Geometry: see drawing. Coordinates: mm, zero at the bounding-box minimum. A direction names the side the tool comes from. Round coordinates to 2 decimals unless told otherwise and drop trailing zeros. Write each loop counter-clockwise with the first axis right and the second up, starting at its lowest first coordinate (ties: lowest second). Pieces come first, ordered by that corner, then holes. Notation, with made-up numbers: M 0,-11 L 58,-11 A23 cw 58,15 Z; hole C 55,16 d3. An arc over 180 degrees is marked long. Write each question's results on one line, items separated by ' | '. Start each with the question number.
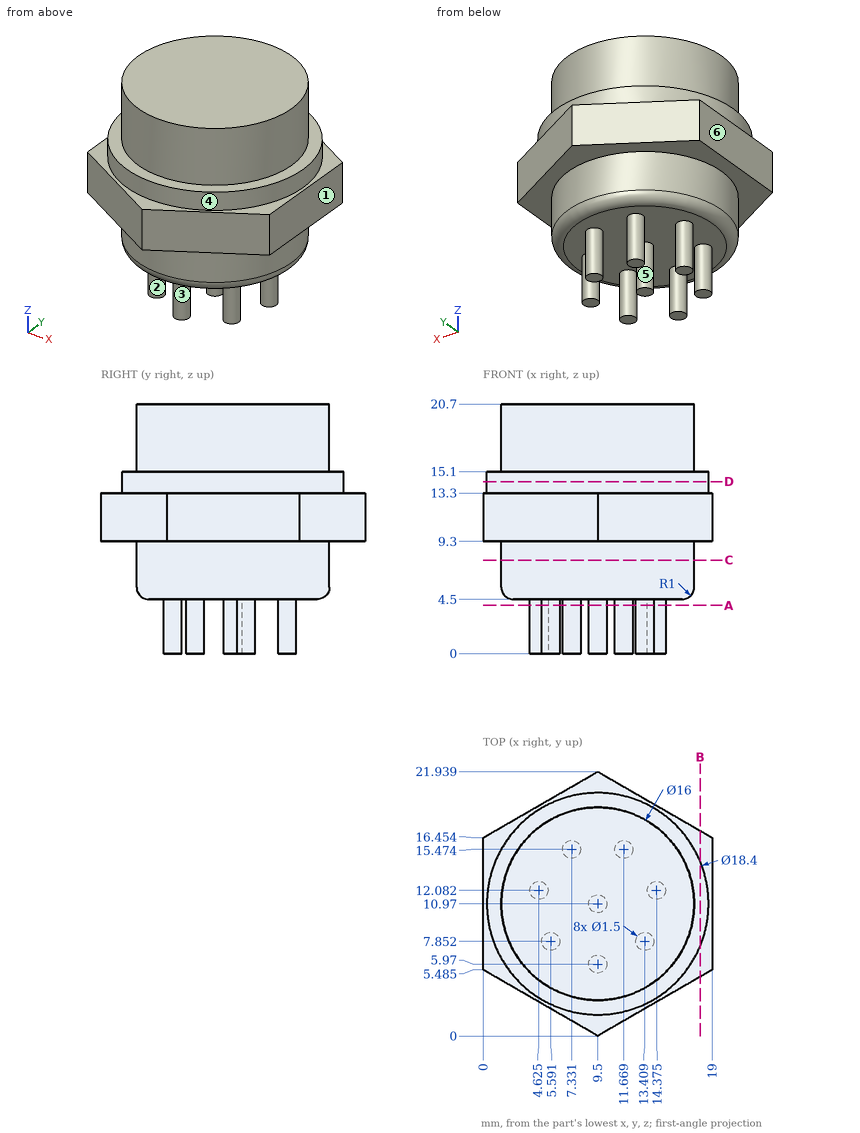
1. Cut plane A-A on z = 4. Give the number of separate pieces and of enclosed holes in the cut face.
2. Access query for the marked faces 4, 5 and 6. Directions: +Z, -Z, +X, -X, +Y, -Y. A direction counts if a zero-diameter tool reaches every point of the face in a straight line with its end or side. Return the directions, or none.
3. Draft query along X for the marked faces 1, 2 and 3. Return one class per face: +X half, -X half, draft (parallel to the pull), parting line (faces both ways), or undercut.
4. Cut plane B-B on x = 18. Output: boundary loops of the cut face in (y, z).
5. Cut plane C-C on z = 7.75. Output: boundary loops of the cut face in (x, y).
6. Line query: L1, parallel to Z at x = 8.5, y = 17; L2, parallel to X at y = 12, z = 2.25; L3, parallel to X at y = 7.25, z = 5.5. Output: solid intervals per line, ascending. Write a range as from..to.
7. Contact query for flat-ended pins moving along their axis: P1, Ø2, axis at x = 3.5, y = 3, coming from the +Z side; P2, Ø10, axis at y = 3.5, z = 3, coming from the -X side; P3, Ø6, axis at x = 2.5, z = 12, coming from the +Y side; P4, Ø5.5, axis at x = 11, y = 6.5, coming from the -Z side. Output: stop coordinate, or through.
8. Cut plane D-D on z = 14.25. Output: boundary loops of the cut face in (x, y), and give its area (3 significant figures).
Answers follow:
1) separate pieces: 8 | enclosed holes: 0
2) face 4: +Z | face 5: -Z | face 6: +Z, -Z, -X, +Y, -Y
3) face 1: +X half | face 2: undercut | face 3: parting line
4) outline: M 4.91,9.3 L 17.03,9.3 L 17.03,13.3 L 14.49,13.3 L 14.49,15.1 L 7.45,15.1 L 7.45,13.3 L 4.91,13.3 Z
5) outline: C 9.5,10.97 d16
6) L1: z = 4.5..20.7 | L2: x = 3.88..5.37, 13.63..15.12 | L3: x = 2.42..16.58
7) P1: stops at z = 15.1 | P2: stops at x = 2.12 | P3: stops at y = 19.63 | P4: stops at z = 0
8) outline: C 9.5,10.97 d18.4 | area: 266 mm2
